Design review of the part built by this model. Coordinates are the model's own, in mm. A direction names the side the tool comes from. Round coordinates to 2 decimals unless told otherwise and drop trailing zeros. Loops run counter-clockwise (first coordinate to the right, second up) from the corner with the lowest first, then second, coordinate; pieces in that order, holes last. Notation, with made-up numbers: (22, 34.5) - (43, 34.5) arc R24 cw to (43, 47.5) - close; hole circle Ø7 at (55, 19). An arc over 180 degrees is marked (long way). Answer as CSV lines item,"result". Start each with the question number.
(1) For P1, Ø1.5, axis at x = 1, z = -2, coming from the -Y side; P2, Ø1, axis at x = 2, y = 1.5, coming from the +Z side (3 decimals); P3, Ø2, axis at x = -1, y = -0.5, coming from the -Z side; P4, Ø1, axis at x = -1, z = 4.5, coming from the -Y side, all flat-tipped, find the tip position at first contact; note any pin that passes through.
(2) Wall thickness on L1, parallel to Z at x = 1.9, y = 0.95 (3 decimals); L2, parallel to Y at x = -1.9, z = -5.25; L3, parallel to X at y = -2.1, z = 2.25: over which ranges is each line inside the solid? List them lowest first.
(3) For faces 3 (the flat face through (0, -2.285, -7)), 4 (the cylindrical face through (-0.415, -0.092, -5.999)), 5 (the cylindrical face through (0.02, -1.38, 6.35)), list the 3-axis set-ups (+Z, -Z, +X, -X, +Y, -Y) from which the entire face can be reached by the end or side of a thin tool; tool diameter is ignored.
(4) Mouldability with a two-part tool opening along Z and no side actions: class faces 1 (the cylindrical face through (0.02, -1.4, -6.35)), 2 (the flat face through (0, -2.285, 7)) as released by +Z, released by -Z, zero draft, split by the parting line, or undercut.
(5) Consider section A-A (x = 0). Give the boundary of the cut face in (y, z) (3 decimals).
(6) Consider section B-B (y = -1.45). Give the boundary of the cut face in (x, z) (3 decimals).
(7) Consider section D-D (y = 0.8). Give the boundary of the cut face in (x, z) (3 decimals), and give its area (3 significant figures).
(8) Consider section C-C (z = 0.25). Give the boundary of the cut face in (x, y) (3 decimals).
from build123d import *

# Parameters (mm, degrees)
SKETCH1_R           = 2.285
BOSS_EXTRUDE1_DEPTH = 5.715
SWEEP1_PROFILE_R    = 0.425


with BuildPart() as part:
    # Sketch1 → Boss-Extrude1 (new, symmetric)
    with BuildSketch(Plane.XY):
        Circle(SKETCH1_R)
    extrude(amount=BOSS_EXTRUDE1_DEPTH, both=True)

    # Sweep1: sweep along a path in Sketch2
    with BuildLine(Plane(origin=(0, 0, 0), x_dir=(0, 0, -1), z_dir=(1, 0, 0))) as sweep1_path:
        Line((-6.775, -2.285), (-6.775, -0.5))
        ThreePointArc((-6.775, -0.5), (-6.628553391, -0.146446609), (-6.275, 0))
        Line((-6.275, 0), (6.275, 0))
        ThreePointArc((6.275, 0), (6.628553391, -0.146446609), (6.775, -0.5))
        Line((6.775, -0.5), (6.775, -2.285))
    # Sweep1 profile (on start of the path) → Sweep1 (sweep)
    with BuildSketch(Plane(origin=(0, -2.285, 6.775), x_dir=(0, 0, 1), z_dir=(0, 1, 0))):
        Circle(SWEEP1_PROFILE_R)
    sweep(path=sweep1_path.line)


solid = part.part
Determined:
1,P1,"stops at y = -2.27"
1,P2,"stops at z = 5.715"
1,P3,"stops at z = -7.2"
1,P4,"stops at y = -2.23"
2,L1,"z = -5.715 to 5.715"
2,L2,"y = -1.27 to 1.27"
2,L3,"x = -0.9 to 0.9"
3,face 3,"+Z, -Z, +X, -X, -Y"
3,face 4,"none"
3,face 5,"-Y"
4,face 1,"undercut"
4,face 2,"zero draft"
5,outline,"(-2.285, -7.2) - (-0.5, -7.2) arc R0.925 ccw to (0.425, -6.275) - (0.425, -5.715) - (2.285, -5.715) - (2.285, 5.715) - (0.425, 5.715) - (0.425, 6.275) arc R0.925 ccw to (-0.5, 7.2) - (-2.285, 7.2) - (-2.285, 6.35) - (-0.5, 6.35) arc R0.075 cw to (-0.425, 6.275) - (-0.425, 5.715) - (-2.285, 5.715) - (-2.285, -5.715) - (-0.425, -5.715) - (-0.425, -6.275) arc R0.075 cw to (-0.5, -6.35) - (-2.285, -6.35) - close"
6,outline,"(-1.766, -5.715) - (1.766, -5.715) - (1.766, 5.715) - (-1.766, 5.715) - close; circle Ø0.85 at (0, -6.775); circle Ø0.85 at (0, 6.775)"
7,outline,"(-2.14, -5.715) - (2.14, -5.715) - (2.14, 5.715) - (-2.14, 5.715) - close"
7,area,"48.9 mm^2"
8,outline,"circle Ø4.57 at (0, 0)"
